Geometry: final body of the model. Coordinates: model frame, mm. A direction names the side the tool comes from. Coordinates: 2 decimals unless noted, no trailing zeros. Write each loop counter-clockwise with the first axis right and the second up, starting at its lowest first coordinate (ties: lowest second). Pieces come first, ordered by that corner, then holes. Notation, with made-up numbers: (-25, 16.5) -> (5, 16.5) arc R33 ccw to (5, 50.5) -> close; hole circle Ø8 at (-19, 22). An arc over 180 degrees is marked (long way). One line per item, written item: value. Start each with the question number.
from build123d import *

# Parameters (mm, degrees)
F1_DEPTH = 9.525
F2_R     = 5.08


# Not quite as in the source:
# - a length typed as a fraction of an inch, garbled in the dataset ("3 / 203.2 mm" for 3/8 in), is restored


with BuildPart() as f1:
    # F0 (on Top) → F1 (new body)
    with BuildSketch(Plane.XY):
        Polygon((19.44, 304.8), (0, 304.8), (-19.44, 304.8), (-19.44, 202.9), (-45.56, 202.9), (-45.56, 304.8), (-68.56, 304.8), (-68.56, 164.8), (-25.4, 164.8), (-25.4, 0), (0, 0), (25.4, 0), (25.4, 164.8), (68.56, 164.8), (68.56, 304.8), (45.56, 304.8), (45.56, 202.9), (19.44, 202.9), align=None)
    extrude(amount=F1_DEPTH)

    # F2
    f2_edges = [f1.edges().sort_by_distance(p)[0] for p in [
        (68.56, 304.8, 4.7625),
        (45.56, 304.8, 4.7625),
        (19.44, 304.8, 4.7625),
        (-19.44, 304.8, 4.7625),
        (-45.56, 304.8, 4.7625),
        (-68.56, 304.8, 4.7625),
        (68.56, 164.8, 4.7625),
        (-25.4, 164.8, 4.7625),
        (-68.56, 164.8, 4.7625),
        (-45.56, 202.9, 4.7625),
        (19.44, 202.9, 4.7625),
        (-19.44, 202.9, 4.7625),
        (45.56, 202.9, 4.7625),
        (25.4, 164.8, 4.7625),
        (25.4, 0, 4.7625),
        (-25.4, 0, 4.7625),
    ]]
    fillet(f2_edges, radius=F2_R)


solid = f1.part
Q1. First-contact query: P1, Ø3, axis at y = 62.5, z = 2.5, coming from the -X side; P2, Ø5, axis at y = 65.5, z = 3, coming from the +X side; P3, Ø3, axis at x = 44.5, z = 6, coming from the -Y side; P4, Ø10, axis at x = -47.5, y = 162.5, coming from the -Z side. Flat tips, straight axial feed; report the tip coordinate or a pass-through.
Q2. Cut plane D-D on y = 26. Output: boundary loops of the cut face in (x, z) (3 decimals).
Q3. Access query for faces 5 (the flat face through (47, 164.8, 5)), 6 (the flat face through (-45.56, 253, 5)), 7 (the flat face through (-57, 304.8, 5)). Directions: +Z, -Z, +X, -X, +Y, -Y. A direction counts if a zero-diameter tool reaches every point of the face in a straight line with its end or side. Return the directions, or none.
Q4. Cut plane C-C on x = -60. Output: boundary loops of the cut face in (y, z) (3 decimals), and give its area (3 significant figures).
Q5. Draft query along X for faces 1 (the cylindrical face through (47.088, 303.351, 4.829)), 2 (the flat face through (68.56, 234, 5)), 3 (the cylindrical face through (-17.912, 303.351, 4.829)), 4 (the flat face through (-25.4, 83, 5)). Return one class per face: pulls with the +X half, pulls with the -X half, needs draft (parallel to the pull), parting line crosses it, or undercut.
Q6. Cut plane A-A on y = 244.5. Output: boundary loops of the cut face in (x, z) (3 decimals).
Q7. Line query: L1, parallel to X at y = 220.5, z = 3; L2, parallel to Y at x = -59, z = 8; L3, parallel to X at y = 115, z = 6.75. Output: solid intervals per line, ascending. Write a range as from..to.
Solution:
1. P1: x = -25.4
1. P2: x = 25.4
1. P3: y = 164.8
1. P4: z = 0
2. outline: (-25.4, 0) -> (25.4, 0) -> (25.4, 9.525) -> (-25.4, 9.525) -> close
3. face 5: +Z, -Z, +X, -Y
3. face 6: +Z, -Z, +Y
3. face 7: +Z, -Z, +X, -X, +Y
4. outline: (164.8, 0) -> (304.8, 0) -> (304.8, 9.525) -> (164.8, 9.525) -> close
4. area: 1,330 mm²
5. face 1: undercut
5. face 2: pulls with the +X half
5. face 3: undercut
5. face 4: pulls with the -X half
6. outline: (-68.56, 0) -> (-45.56, 0) -> (-45.56, 9.525) -> (-68.56, 9.525) -> close; (-19.44, 0) -> (19.44, 0) -> (19.44, 9.525) -> (-19.44, 9.525) -> close; (45.56, 0) -> (68.56, 0) -> (68.56, 9.525) -> (45.56, 9.525) -> close
7. L1: -68.56..-45.56, -19.44..19.44, 45.56..68.56
7. L2: 164.8..304.8
7. L3: -25.4..25.4
